from build123d import *
from build123d import SkipClean  # not in build123d's __all__

# Parameters (mm, degrees)
F0_R      = 1.6
F0_R_2    = 8.25
F0_R_3    = 3
F1_DEPTH  = 3
F2_R      = 3
F2_R_2    = 1.6
F2_R_3    = 8.25
F3_DEPTH  = 34
F4_W      = 30.5
F4_H      = 30.5
F5_DEPTH  = 5
F6_W      = 27.5
F6_H      = 28.5
F7_DEPTH  = 24.77
F9_DEPTH  = 32
F10_R     = 1.6
F11_DEPTH = 39.001
F12_R     = 1.6
F13_DEPTH = 2
F15_DEPTH = 4
F16_R     = 1.6
F17_DEPTH = 4
F20_R     = 1.2
F21_DEPTH = 5
F22_R     = 1
F23_DEPTH = 9.591955051
F25_DEPTH = 2.342955051


# Not quite as in the source:
# - after a boolean that leaves OpenCascade's solid faulty, fix() repairs it


with BuildPart() as f1:
    # F0 (on Top) → F1 (new body)
    with BuildSketch(Plane.XY):
        Polygon((-25, 29), (-25, 0), (-16.091955051, 0), (-16.091955051, -4), (16.091955051, -4), (16.091955051, 0), (25, 0), (25, 29), (19, 35), (-19, 35), align=None)
        with Locations((-10.5, 8.4)):
            Circle(F0_R, mode=Mode.SUBTRACT)
        with Locations((10.5, 8.4)):
            Circle(F0_R, mode=Mode.SUBTRACT)
        with Locations((0, 14.5)):
            Circle(F0_R_2, mode=Mode.SUBTRACT)
        with Locations((-8.75, 25.5)):
            Circle(F0_R_3, mode=Mode.SUBTRACT)
        with Locations((0, 26.6)):
            Circle(F0_R, mode=Mode.SUBTRACT)
        with Locations((8.75, 25.5)):
            Circle(F0_R_3, mode=Mode.SUBTRACT)
    extrude(amount=F1_DEPTH)

    # F2 (on face) → F3 (join)
    with BuildSketch(Plane(origin=(0, 0, 0), x_dir=(1, 0, 0), z_dir=(0, 0, -1))):
        Polygon((16.091955051, 4), (-16.091955051, 4), (-16.091955051, 0), (-16.091955051, -35), (16.091955051, -35), (16.091955051, 0), align=None)
        with Locations((-8.75, -25.5)):
            Circle(F2_R, mode=Mode.SUBTRACT)
        with Locations((0, -26.6)):
            Circle(F2_R_2, mode=Mode.SUBTRACT)
        with Locations((8.75, -25.5)):
            Circle(F2_R, mode=Mode.SUBTRACT)
        with Locations((-10.5, -8.4)):
            Circle(F2_R_2, mode=Mode.SUBTRACT)
        with Locations((0, -14.5)):
            Circle(F2_R_3, mode=Mode.SUBTRACT)
        with Locations((10.5, -8.4)):
            Circle(F2_R_2, mode=Mode.SUBTRACT)
    extrude(amount=F3_DEPTH)

    # F4 (on face) → F5 (cut)
    with BuildSketch(Plane(origin=(0, 35, 0), x_dir=(-1, 0, 0), z_dir=(0, 1, 0))):
        with Locations((-0.091955051, -15.25)):
            Rectangle(F4_W, F4_H)
    extrude(amount=-F5_DEPTH, mode=Mode.SUBTRACT)

    # F6 (on face) → F7 (cut)
    with BuildSketch(Plane(origin=(0, 30, 0), x_dir=(-1, 0, 0), z_dir=(0, 1, 0))):
        with Locations((0, -16.25)):
            Rectangle(F6_W, F6_H)
    extrude(amount=-F7_DEPTH, mode=Mode.SUBTRACT)

    # F8 (on face) → F9 (cut)
    with BuildSketch(Plane(origin=(0, 0, -34), x_dir=(1, 0, 0), z_dir=(0, 0, -1))):
        with BuildLine():
            Line((8.25, -14.5), (13.5, -14.5))
            ThreePointArc((13.5, -14.5), (13.1444351182, -11.4220420042), (12.0964703076, -8.5062193819))
            ThreePointArc((12.0964703076, -8.5062193819), (9.1165222882, -9.2037346707), (11.1984910379, -6.9605173603))
            ThreePointArc((11.1984910379, -6.9605173603), (0, -1), (-11.1984910379, -6.9605173603))
            ThreePointArc((-11.1984910379, -6.9605173603), (-9.6507608289, -7.043979045), (-8.9, -8.4))
            ThreePointArc((-8.9, -8.4), (-10.4468609941, -9.9991173334), (-12.0964703076, -8.5062193819))
            ThreePointArc((-12.0964703076, -8.5062193819), (-13.1444351182, -11.4220420042), (-13.5, -14.5))
            Line((-13.5, -14.5), (-8.25, -14.5))
            ThreePointArc((-8.25, -14.5), (0, -6.25), (8.25, -14.5))
        make_face()
        with BuildLine():
            Line((13.5, -35), (13.5, -14.5))
            ThreePointArc((13.5, -14.5), (12.717238531, -19.0301042091), (10.4597267933, -23.0348764144))
            ThreePointArc((10.4597267933, -23.0348764144), (11.4079296812, -24.1088099303), (11.75, -25.5))
            ThreePointArc((11.75, -25.5), (9.3158770477, -28.4461471733), (5.9634778888, -26.611438043))
            ThreePointArc((5.9634778888, -26.611438043), (3.4585284768, -27.5494666855), (0.8178060745, -27.9752066116))
            ThreePointArc((0.8178060745, -27.9752066116), (0, -28.2), (-0.8178060745, -27.9752066116))
            ThreePointArc((-0.8178060745, -27.9752066116), (-3.4585284768, -27.5494666855), (-5.9634778888, -26.611438043))
            ThreePointArc((-5.9634778888, -26.611438043), (-10.6175706975, -27.8478031625), (-10.4597267933, -23.0348764144))
            ThreePointArc((-10.4597267933, -23.0348764144), (-12.717238531, -19.0301042091), (-13.5, -14.5))
            Line((-13.5, -14.5), (-13.5, -35))
            Line((-13.5, -35), (13.5, -35))
        make_face()
        with BuildLine():
            ThreePointArc((10.4597267933, -23.0348764144), (12.717238531, -19.0301042091), (13.5, -14.5))
            Line((13.5, -14.5), (8.25, -14.5))
            ThreePointArc((8.25, -14.5), (0, -22.75), (-8.25, -14.5))
            Line((-8.25, -14.5), (-13.5, -14.5))
            ThreePointArc((-13.5, -14.5), (-12.717238531, -19.0301042091), (-10.4597267933, -23.0348764144))
            ThreePointArc((-10.4597267933, -23.0348764144), (-7.3588099303, -22.8420703188), (-5.75, -25.5))
            ThreePointArc((-5.75, -25.5), (-5.8038528267, -26.0658770477), (-5.9634778888, -26.611438043))
            ThreePointArc((-5.9634778888, -26.611438043), (-3.4585284768, -27.5494666855), (-0.8178060745, -27.9752066116))
            ThreePointArc((-0.8178060745, -27.9752066116), (-0.7910468636, -25.2092286818), (1.6, -26.6))
            ThreePointArc((1.6, -26.6), (1.3907713182, -27.3910468636), (0.8178060745, -27.9752066116))
            ThreePointArc((0.8178060745, -27.9752066116), (3.4585284768, -27.5494666855), (5.9634778888, -26.611438043))
            ThreePointArc((5.9634778888, -26.611438043), (6.8824293025, -23.1521968375), (10.4597267933, -23.0348764144))
        make_face()
        with BuildLine():
            ThreePointArc((11.1984910379, -6.9605173603), (9.1165222882, -9.2037346707), (12.0964703076, -8.5062193819))
            ThreePointArc((12.0964703076, -8.5062193819), (11.6730931936, -7.7184887161), (11.1984910379, -6.9605173603))
        make_face()
    extrude(amount=-F9_DEPTH, mode=Mode.SUBTRACT)

    # F10 (on face) → F11 (cut, through all)
    with BuildSketch(Plane.XZ.offset(4)):
        with Locations((-11.091955051, -5.5)):
            Circle(F10_R)
        Polygon((-3.5, -3.5), (-6.5, -6.5), (-6.5, -27.5), (-3.5, -30.5), (3.5, -30.5), (6.5, -27.5), (6.5, -6.5), (3.5, -3.5), align=None)
        with Locations((-11.091955051, -17.5)):
            Circle(F10_R)
        with Locations((11.091955051, -17.5)):
            Circle(F10_R)
        with Locations((11.091955051, -5.5)):
            Circle(F10_R)
    extrude(amount=-F11_DEPTH, mode=Mode.SUBTRACT)

    # F12 (on face) → F13 (cut)
    with BuildSketch(Plane(origin=(0, 0, -2), x_dir=(1, 0, 0), z_dir=(0, 0, -1))):
        Polygon((-8.8689854895, -11.225), (-7.2379709791, -8.4), (-8.8689854895, -5.575), (-12.1310145105, -5.575), (-13.75, -8.3791651246), (-13.75, -8.4208348754), (-12.1310145105, -11.225), align=None)
        with Locations((-10.5, -8.4)):
            Circle(F12_R, mode=Mode.SUBTRACT)
        Polygon((12.1310145105, -11.225), (13.75, -8.4208348754), (13.75, -8.3791651246), (12.1310145105, -5.575), (8.8689854895, -5.575), (7.2379709791, -8.4), (8.8689854895, -11.225), align=None)
        with Locations((10.5, -8.4)):
            Circle(F12_R, mode=Mode.SUBTRACT)
        Polygon((1.6310145105, -29.425), (3.2620290209, -26.6), (1.6310145105, -23.775), (-1.6310145105, -23.775), (-3.2620290209, -26.6), (-1.6310145105, -29.425), align=None)
        with Locations((0, -26.6)):
            Circle(F12_R, mode=Mode.SUBTRACT)
    extrude(amount=-F13_DEPTH, mode=Mode.SUBTRACT)

    # F14 (on face) → F15 (join)
    with BuildSketch(Plane(origin=(0, 0, -2), x_dir=(1, 0, 0), z_dir=(0, 0, -1))):
        with BuildLine():
            Line((-13.75, -30), (-9.25, -30))
            Line((-9.25, -30), (-9.25, -28.4580398915))
            ThreePointArc((-9.25, -28.4580398915), (-11.1952034569, -27.2380966757), (-11.7080398915, -25))
            Line((-11.7080398915, -25), (-13.75, -25))
            Line((-13.75, -25), (-13.75, -30))
        make_face()
        with BuildLine():
            Line((9.25, -30), (13.75, -30))
            Line((13.75, -30), (13.75, -25))
            Line((13.75, -25), (11.7080398915, -25))
            ThreePointArc((11.7080398915, -25), (11.7394915684, -25.2491212192), (11.75, -25.5))
            ThreePointArc((11.75, -25.5), (11.0412878475, -27.4364916731), (9.25, -28.4580398915))
            Line((9.25, -28.4580398915), (9.25, -30))
        make_face()
    with SkipClean():  # cleaning this boolean's faces spoils the solid; the shape is the same uncleaned
        extrude(amount=F15_DEPTH)


with BuildPart() as f17:
    # F16 (on face) → F17 (new body)
    with BuildSketch(Plane.XZ.offset(4)):
        Polygon((-11.091955051, -8.7620290209), (-8.266955051, -7.1310145105), (-8.266955051, -3.8689854895), (-11.091955051, -2.2379709791), (-13.916955051, -3.8689854895), (-13.916955051, -7.1310145105), align=None)
        with Locations((-11.091955051, -5.5)):
            Circle(F16_R, mode=Mode.SUBTRACT)
    extrude(amount=F17_DEPTH)


with BuildPart() as f17b:
    # F16 (on face) → F17, piece 2 (new body)
    with BuildSketch(Plane.XZ.offset(4)):
        Polygon((-11.091955051, -20.7620290209), (-8.266955051, -19.1310145105), (-8.266955051, -15.8689854895), (-11.091955051, -14.2379709791), (-13.916955051, -15.8689854895), (-13.916955051, -19.1310145105), align=None)
        with Locations((-11.091955051, -17.5)):
            Circle(F16_R, mode=Mode.SUBTRACT)
    extrude(amount=F17_DEPTH)


with BuildPart() as f17c:
    # F16 (on face) → F17, piece 3 (new body)
    with BuildSketch(Plane.XZ.offset(4)):
        Polygon((11.091955051, -20.7620290209), (13.916955051, -19.1310145105), (13.916955051, -15.8689854895), (11.091955051, -14.2379709791), (8.266955051, -15.8689854895), (8.266955051, -19.1310145105), align=None)
        with Locations((11.091955051, -17.5)):
            Circle(F16_R, mode=Mode.SUBTRACT)
    extrude(amount=F17_DEPTH)


with BuildPart() as f17d:
    # F16 (on face) → F17, piece 4 (new body)
    with BuildSketch(Plane.XZ.offset(4)):
        Polygon((11.091955051, -8.7620290209), (13.916955051, -7.1310145105), (13.916955051, -3.8689854895), (11.091955051, -2.2379709791), (8.266955051, -3.8689854895), (8.266955051, -7.1310145105), align=None)
        with Locations((11.091955051, -5.5)):
            Circle(F16_R, mode=Mode.SUBTRACT)
    extrude(amount=F17_DEPTH)


with BuildPart() as f17_1:
    # F18: moved
    add(f17.part.moved(Location((0, 10.3, 0))), clean=False)


with BuildPart() as f17b_1:
    # F18: moved
    add(f17b.part.moved(Location((0, 10.3, 0))), clean=False)


with BuildPart() as f17d_1:
    # F18: moved
    add(f17d.part.moved(Location((0, 10.3, 0))), clean=False)


with BuildPart() as f17c_1:
    # F18: moved
    add(f17c.part.moved(Location((0, 10.3, 0))), clean=False)


with BuildPart() as f1_1:
    add(f1.part, clean=False)

    # F19: cut F17, F17b, F17d, F17c
    add(f17_1.part, mode=Mode.SUBTRACT)
    add(f17b_1.part, mode=Mode.SUBTRACT)
    add(f17d_1.part, mode=Mode.SUBTRACT)
    add(f17c_1.part, mode=Mode.SUBTRACT)

    add(f1_1.part.fix(), mode=Mode.REPLACE)

    # F20 (on face) → F21 (cut, through all)
    with BuildSketch(Plane(origin=(0, 30, 0), x_dir=(-1, 0, 0), z_dir=(0, 1, 0))):
        with Locations((-12, -3.25)):
            Circle(F20_R)
        with Locations((12, -3.25)):
            Circle(F20_R)
    extrude(amount=-F21_DEPTH, mode=Mode.SUBTRACT)

    # F22 (on face) → F23 (cut, through all)
    with BuildSketch(Plane(origin=(-16.091955051, 0, 0), x_dir=(0, -1, 0), z_dir=(-1, 0, 0))):
        with Locations((-1, -26)):
            Circle(F22_R)
    extrude(amount=-F23_DEPTH, mode=Mode.SUBTRACT)

    # F24 (on face) → F25 (cut, through all)
    with BuildSketch(Plane.YZ.offset(16.091955051)):
        with BuildLine():
            ThreePointArc((30, -27), (30.7071067812, -26.7071067812), (31, -26))
            ThreePointArc((31, -26), (30.7071067812, -25.2928932188), (30, -25))
            Line((30, -25), (30, -27))
        make_face()
        with BuildLine():
            Line((30, -27), (30, -25))
            ThreePointArc((30, -25), (29, -26), (30, -27))
        make_face()
        with BuildLine():
            ThreePointArc((30, -25), (30.7071067812, -25.2928932188), (31, -26))
            ThreePointArc((31, -26), (30.7071067812, -26.7071067812), (30, -27))
            Line((30, -27), (33, -27))
            ThreePointArc((33, -27), (32, -26), (33, -25))
            Line((33, -25), (30, -25))
        make_face()
        with BuildLine():
            ThreePointArc((34, -26), (33.7071067812, -25.2928932188), (33, -25))
            Line((33, -25), (33, -27))
            ThreePointArc((33, -27), (33.7071067812, -26.7071067812), (34, -26))
        make_face()
        with BuildLine():
            Line((33, -27), (33, -25))
            ThreePointArc((33, -25), (32, -26), (33, -27))
        make_face()
    extrude(amount=-F25_DEPTH, mode=Mode.SUBTRACT)


solid = f1_1.part
For this review, take the finished solid that the model builds, in its own axes (mm). A direction names the side the tool comes from. Coordinates: 2 decimals unless noted, no trailing zeros. Loops run counter-clockwise (first coordinate to the right, second up) from the corner with the lowest first, then second, coordinate; pieces in that order, holes last. Notation, with made-up numbers: (71, 53) - (96, 53) arc R25 ccw to (96, 79) - close; hole circle Ø7 at (85.5, -30.5). An arc over 180 degrees is marked (long way). Use a Markdown table: item, result. Add a question column.
Item 1: Tool access review of faces 5 (the face through (9.32, 7.32, 1.52)), 6 (the face through (15, 30, -29)), 7 (the face through (8.04, 9.79, -1.01)), 8 (the face through (12, 2.3, -4)), 9 (the face through (0, -1, -30.5)): name each direction out of +Z, -Z, +X, -X, +Y, -Y from which nothing blocks a thin tool from reaching the whole face with its end or side.
Item 2: We need section D-D (y = 21.5). Give the boundary of the cut face in (x, z).
Item 3: Mouldability with a two-part tool opening along Y and no side actions: class faces 1 (the face through (10, 11.225, -1)), 2 (the face through (-16.092, 15, -15)), 3 (the face through (0, 23.775, -1)), 4 (the face through (-12, 5.23, -25)) as pulls with the +Y half, pulls with the -Y half, needs draft (parallel to the pull), parting line crosses it, or undercut.
Item 4: We need section C-C (z = -28.5). Give the boundary of the cut face in (x, y).
Item 5: For line 1 (X direction, y = 25.5, z = -0.55); line 2 (X direction, y = 32, z = -12); line 3 (X direction, y = 8, z = 2), list the stretches that pass through material, from the lowest coordinate up.
Item 6: Insertion check: pin 1 Ø3 at (y, z) = (1, -26) entering from +X; pin 2 Ø3 at (x, z) = (11, -18) entering from +Y; pin 3 Ø2 at (x, z) = (11, -1.5) entering from +Y. Each pin has a flat end and moves straight along its axis. Give the tip position at first contact, or say it passes through.
Item 7: We need section B-B (x = 0). Give the boundary of the cut face in (y, z) (3 decimals).
Item 8: We need section A-A (y = 32). Give the boundary of the cut face in (x, z).
Results list:
| question | item | result |
|---|---|---|
| 1 | face 5 | +Z, -Z |
| 1 | face 6 | +Y |
| 1 | face 7 | -Z |
| 1 | face 8 | none |
| 1 | face 9 | +Y, -Y |
| 2 | outline | (-25, 0) - (-16.09, 0) - (-16.09, -34) - (-13.5, -34) - (-13.5, -30.5) - (-13.75, -30.5) - (-13.75, -2) - (-4.37, -2) - (-4.37, 3) - (-25, 3) - close; (4.37, -2) - (13.75, -2) - (13.75, -30.5) - (13.5, -30.5) - (13.5, -34) - (16.09, -34) - (16.09, 0) - (25, 0) - (25, 3) - (4.37, 3) - close |
| 3 | face 1 | undercut |
| 3 | face 2 | needs draft |
| 3 | face 3 | undercut |
| 3 | face 4 | pulls with the +Y half |
| 4 | outline | (-16.09, -4) - (-5.5, -4) - (-5.5, 2.17) arc R13.5 cw to (-9.81, 5.23) - (-13.75, 5.23) - (-13.75, 30) - (-15.16, 30) - (-15.16, 35) - (-16.09, 35) - close; (5.5, -4) - (16.09, -4) - (16.09, 35) - (15.34, 35) - (15.34, 30) - (13.75, 30) - (13.75, 5.23) - (9.81, 5.23) arc R13.5 cw to (5.5, 2.17) - close |
| 5 | line 1 | x = -16.09 to -11.75, -5.75 to -2.63, 2.63 to 5.75, 11.75 to 16.09 |
| 5 | line 2 | x = -16.09 to -15.16, 15.34 to 16.09 |
| 5 | line 3 | x = -25 to -12.05, -8.95 to -5.08, 5.08 to 8.95, 12.05 to 25 |
| 6 | pin 1 | stops at x = 16.09 |
| 6 | pin 2 | stops at y = 2.3 |
| 6 | pin 3 | stops at y = 30 |
| 7 | outline | (-4, -34) - (1, -34) - (1, -30.5) - (-4, -30.5) - close; (-4, -3.5) - (1, -3.5) - (1, -2) - (6.25, -2) - (6.25, 3) - (-4, 3) - close; (22.75, -2) - (23.775, -2) - (23.775, 0) - (25, 0) - (25, 3) - (22.75, 3) - close; (28.2, 0) - (29.425, 0) - (29.425, -2) - (30, -2) - (30, 0) - (35, 0) - (35, 3) - (28.2, 3) - close |
| 8 | outline | (-22, 0) - (-16.09, 0) - (-16.09, -34) - (-13.5, -34) - (-13.5, -30.5) - (-15.16, -30.5) - (-15.16, 0) - (15.34, 0) - (15.34, -25) - (16.09, -25) - (16.09, 0) - (22, 0) - (22, 3) - (-22, 3) - close; (13.5, -34) - (16.09, -34) - (16.09, -27) - (15.34, -27) - (15.34, -30.5) - (13.5, -30.5) - close |
